Check sheet for the drawn part. Datum: minimum x, y, z corner. Units: mm. Round coordinates to 2 decimals unless told otherwise and drop trailing zeros. Write each loop counter-clockwise with the first axis right and the second up, starting at its lowest first coordinate (ties: lowest second). Pieces come first, ordered by that corner, then holes. Notation, with made-up numbers: M 49,39 L 53,39 A4 cw 53,43 Z; hole C 12.25,60.5 d8. An arc over 180 degrees is marked long. One line per item, written item: value. Start each with the question number.
1. Release check for a two-part mould opening along X. For the marked faces 1, 2 and 3 record: pulls with the +X half, pulls with the -X half, needs draft (parallel to the pull), parting line crosses it, or undercut.
2. Section check B-B (x = 6.35). Record the boundary of the cut face in (y, z), and give its area (3 significant figures).
3. Section check C-C (y = 0.4). Record the boundary of the cut face in (x, z).
4. Section check A-A (z = 8.89). Record the boundary of the cut face in (x, y).
5. Depth check by flat-ended pin: P1, Ø1.5, axis at x = 6.35, z = 8.89, coming from the -Y side. Enter the tip coordinate at first touch or a pass-through.
6. Section check D-D (z = 3.81). Record the boundary of the cut face in (x, y), and give its area (3 significant figures).
7. Scan lines: probe 1 along X at (y, z) = (0.6, 3.81); probe 2 along Z at (x, y) = (6.75, 2.2); probe 3 along X at (y, z) = (1.45, 8.89). Record each from-to range of solid material in increasing order. Write a range as [from, to].
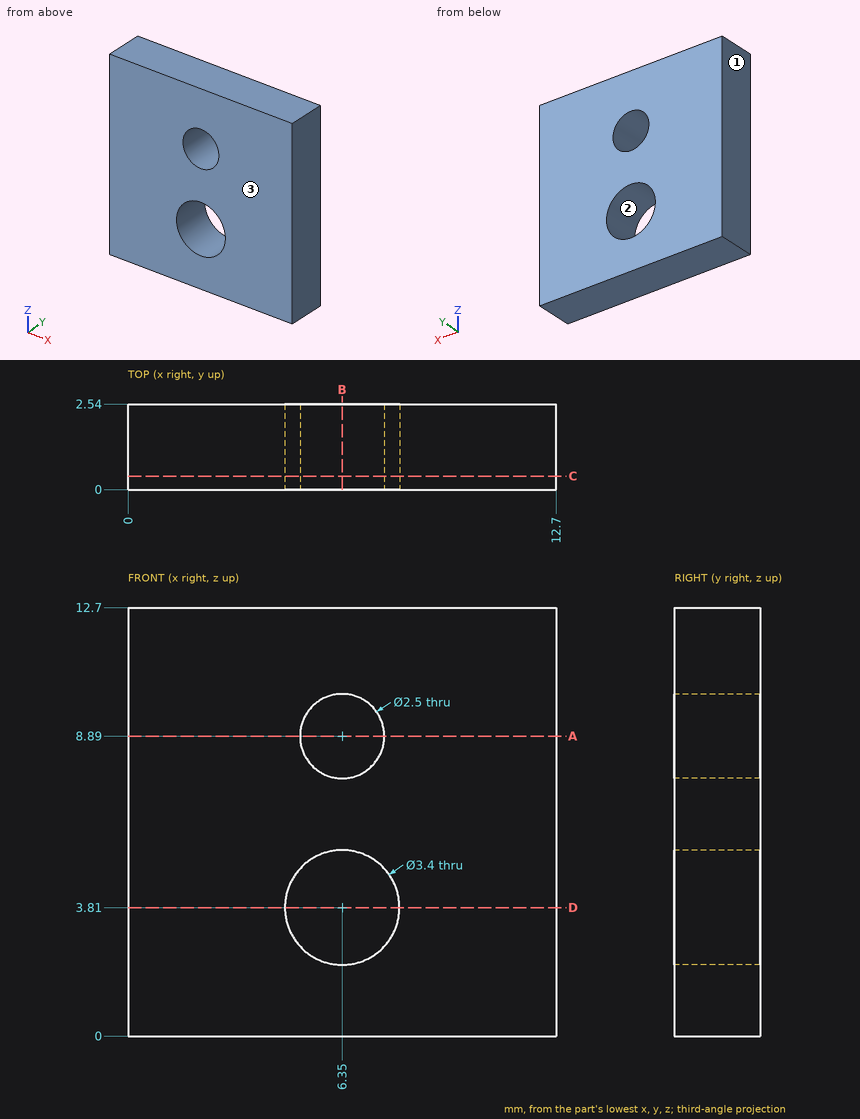
Result sheet:
1. face 1: pulls with the -X half
1. face 2: undercut
1. face 3: needs draft
2. outline: M 0,0 L 2.54,0 L 2.54,2.11 L 0,2.11 Z; M 0,5.51 L 2.54,5.51 L 2.54,7.64 L 0,7.64 Z; M 0,10.14 L 2.54,10.14 L 2.54,12.7 L 0,12.7 Z
2. area: 17.3 mm2
3. outline: M 0,0 L 12.7,0 L 12.7,12.7 L 0,12.7 Z; hole C 6.35,3.81 d3.4; hole C 6.35,8.89 d2.5
4. outline: M 0,0 L 5.1,0 L 5.1,2.54 L 0,2.54 Z; M 7.6,0 L 12.7,0 L 12.7,2.54 L 7.6,2.54 Z
5. P1: passes through
6. outline: M 0,0 L 4.65,0 L 4.65,2.54 L 0,2.54 Z; M 8.05,0 L 12.7,0 L 12.7,2.54 L 8.05,2.54 Z
6. area: 23.6 mm2
7. probe 1: x = [0, 4.65], [8.05, 12.7]
7. probe 2: z = [0, 2.16], [5.46, 7.71], [10.07, 12.7]
7. probe 3: x = [0, 5.1], [7.6, 12.7]
